Geometry: see drawing. Coordinates: mm, zero at the bounding-box minimum. Round coordinates to 2 decimals unless told otherwise and drop trailing zeros. Loops run counter-clockwise (first coordinate to the right, second up) from the corner with the lowest first, then second, coordinate; pieces in that order, holes last. Notation, with made-up numbers: (40.5, -16.5) - (86.5, -16.5) arc R31 cw to (86.5, 15.5) - close; hole circle Ø9 at (40, 24). An arc over 180 degrees is marked (long way). Use CSV: the item, a comma, the result in double quotes. Start each with the question number.
1. Cut plane A-A (x = 37.5). Return loops of the section in (y, z).
2. Cut plane C-C (z = 2.75). Give the number of separate pieces and of enclosed holes in the cut face, and give its area (3 significant figures).
3. Pin query (flat end, axial travel): P1, Ø3, axis at x = 20.5, y = 70.5, coming from the +Z side; P2, Ø7, axis at x = 145, z = 7.5, coming from the +Y side; P3, Ø2, axis at y = 52, z = 7.5, coming from the +X side (1 decimal); P4, Ø1, axis at x = 103.5, z = 3, coming from the -Y side. Return the tip coordinate at first contact, or that it passes through.
4. Pull-direction query (Y, two-part tool) for the marked faces 1, 2, 3 and 4; classes: +Y half, -Y half, draft (parallel to the pull), parting line (faces both ways), or undercut.
5. Material intervals for probe 1 along X at (y, z) = (29.5, 2.75) (1 decimal); probe 2 along X at (y, z) = (36.5, 13.25); probe 3 along Y at (x, z) = (12.5, 2) (1 decimal), sorted ascending. Write a range as from..to.
6. Cut plane D-D (x = 145). Return loops of the section in (y, z).
7. Cut plane B-B (y = 45). Return loops of the section in (x, z), and give its area (3 significant figures).
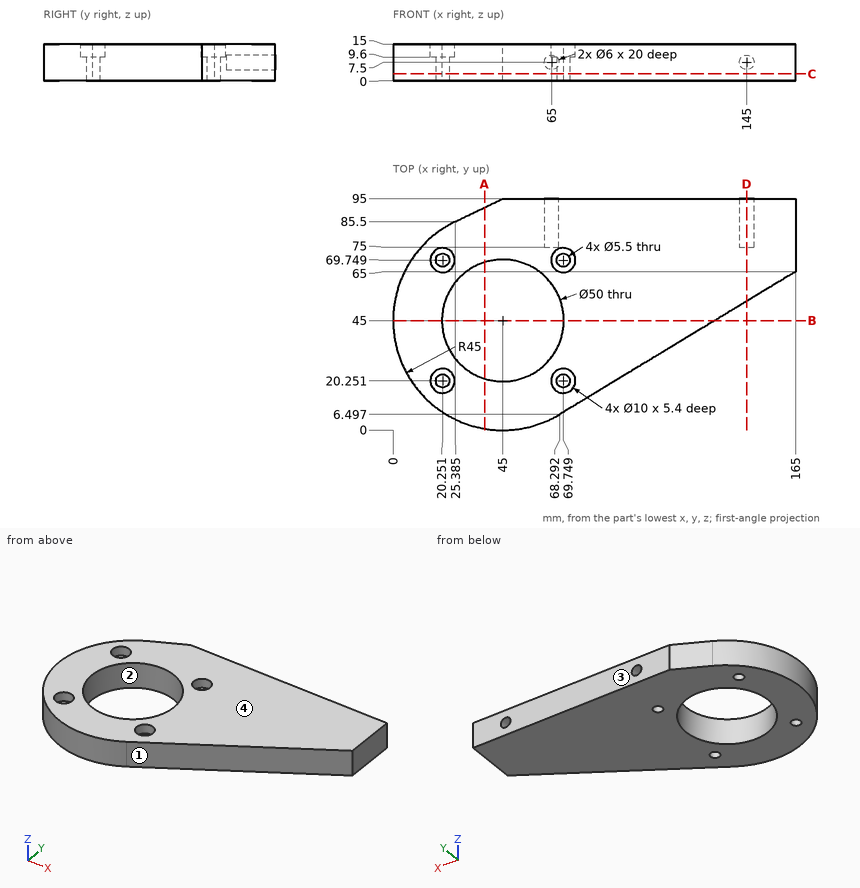
Established:
1,outline,"(0.63, 0) - (21.15, 0) - (21.15, 15) - (0.63, 15) - close; (68.85, 0) - (91.37, 0) - (91.37, 15) - (68.85, 15) - close"
2,separate pieces,"1"
2,enclosed holes,"5"
2,area,"9,050 mm2"
3,P1,"passes through"
3,P2,"stops at y = 95"
3,P3,"stops at x = 145.2"
3,P4,"stops at y = 27.49"
4,face 1,"-Y half"
4,face 2,"undercut"
4,face 3,"+Y half"
4,face 4,"draft"
5,probe 1,"x = 2.8..25.4, 64.6..106.3"
5,probe 2,"x = 0.81..21.49, 68.51..117.89"
5,probe 3,"y = 13.9..76.1"
6,outline,"(52.9, 0) - (95, 0) - (95, 4.5) - (75, 4.5) - (75, 10.5) - (95, 10.5) - (95, 15) - (52.9, 15) - close"
7,outline,"(0, 0) - (20, 0) - (20, 15) - (0, 15) - close; (70, 0) - (131.94, 0) - (131.94, 15) - (70, 15) - close"
7,area,"1,230 mm2"
